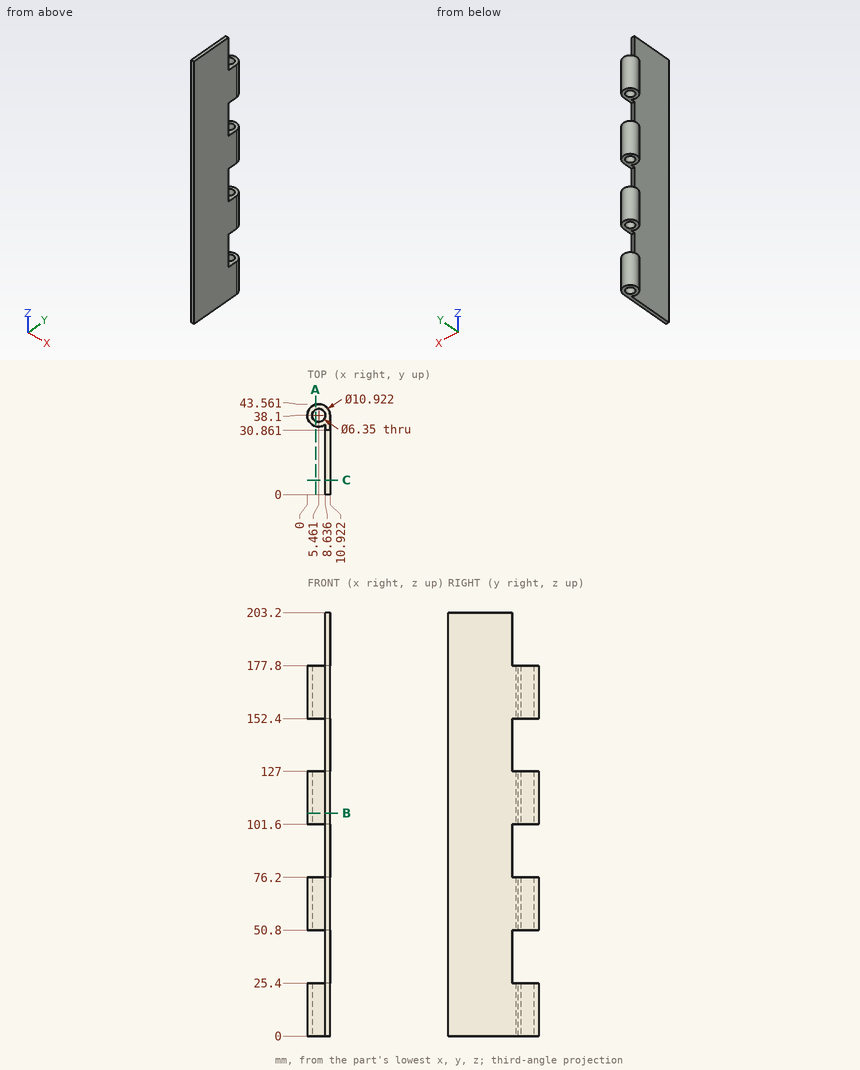
Answer from the drawing. Dimensions are ordinates in mm from the lowest x, y and z of the part. Round coordinates to 2 decimals unless told otherwise and drop trailing zeros. Loops run counter-clockwise (first coordinate to the right, second up) from the corner with the lowest first, then second, coordinate; pieces in that order, holes last.
(1) Each of these flat-tipped pins is pushed along its axis until it touches: P1, Ø1.1, axis at x = 9.5, z = 188, coming from the +Y side; P2, Ø1.5, axis at y = 23.5, z = 174, coming from the -X side; P3, Ø3.5, axis at x = 7, y = 35, coming from the +Z side. Where does it stop, or does it pass through?
Computed values:
P1: stops at y = 30.86
P2: stops at x = 8.64
P3: stops at z = 177.8
(2) The part is cut by section A-A, the plane x = 4. Give the number of separate pieces and of enclosed holes in the cut face, and give its area (3 significant figures).
Computed values:
separate pieces: 8
enclosed holes: 0
area: 496 mm2
(3) The part is cut by section B-B, the plane z = 107. Give the vertices of the cut face in (x, y) (3 decimals).
Computed values:
outline: (8.636, 0) - (10.922, 0) - (10.922, 38.1) arc R5.461 ccw (long way) to (8.636, 33.657) - close; hole circle Ø6.35 at (5.461, 38.1)
(4) Find the intervals of material crossed by L1, parallel to Z at x = 4, y = 33; L2, parallel to X at y = 38.1, z = 11.5; L3, parallel to X at y = 19.5, z = 162, in increasing order.
Computed values:
L1: z = 0 to 25.4, 50.8 to 76.2, 101.6 to 127, 152.4 to 177.8
L2: x = 0 to 2.29, 8.64 to 10.92
L3: x = 8.64 to 10.92
(5) The part is cut by section C-C, the plane y = 7. Give the vertices of the cut face in (x, z).
Computed values:
outline: (8.64, 0) - (10.92, 0) - (10.92, 203.2) - (8.64, 203.2) - close
